The model under review builds one solid part; all positions refer to its coordinate system, in mm. A direction names the side the tool comes from. Coordinates: 2 decimals unless noted, no trailing zeros. Loops run counter-clockwise (first coordinate to the right, second up) from the corner with the lowest first, then second, coordinate; pieces in that order, holes last. Notation, with made-up numbers: M 49.25,-24.75 L 108.25,-24.75 A19 ccw 108.25,-0.75 Z; hole C 57.25,80.25 d6. An arc over 180 degrees is marked long. Use CSV: the item, a comma, the result in double quotes. Start each with the question number.
1. Add section C-C, the plane y = 12.5. Write out the cut boundary in (x, z), then the cut area to 3 significant figures.
2. Tool access review of faces 4 (the cylindrical face through (-68.092, 50.041, 19.399)), 5 (the flat face through (1, 0, 10)), 6 (the flat face through (1, 24, 0)): name each direction out of +Z, -Z, +X, -X, +Y, -Y from which nothing blocks a thin tool from reaching the whole face with its end or side.
3. Add section A-A, the plane z = 34. Write out the cut boundary in (x, y).
4. Clearance check with flat-ended pins moving along their axes: P1, Ø6.5, axis at x = 31.5, z = 20, coming from the -Y side; P2, Ø5, axis at x = 70, z = 20, coming from the -Y side; P3, Ø2.5, axis at x = -70, z = 20, coming from the -Y side. State where each tip first meets the part, or that it passes through.
5. For L1, parallel to Z at x = 80, y = 5; L2, parallel to X at y = 35, z = 36.5; L3, parallel to X at y = 25, z = 20, list the stretches that pass through material, from the lowest coordinate up.
6. Add section B-B, the plane x = -31.5. Write out the cut boundary in (y, z), then the cut area to 3 significant figures.
7. Add section D-D, the plane z = 20. Write out the cut boundary in (x, y), then the cut area to 3 significant figures.
8. Draft analysis for pull direction Z (two halves, no side actions). For faces 1 (the flat face through (1, 25, 40)), 2 (the flat face through (1, -5.303, 5)), 3 (the cylindrical face through (31.17, 34.26, 17.52)), state which applies: +Z half, -Z half, draft (parallel to the pull), parting line (faces both ways), or undercut.
from build123d import *

# Parameters (mm, degrees)
SKETCH1_R                       = 10.75
BOSS_EXTRUDE1_DEPTH             = 40
BOSS_EXTRUDE2_REACH             = 92
BOSS_EXTRUDE2_DIRECTION_2_REACH = 92
SKETCH5_R                       = 2.5
CUT_EXTRUDE1_DEPTH              = 54.696523
CUT_EXTRUDE3_REACH              = 62
SKETCH8_R                       = 2


with BuildPart() as part:
    # Sketch1 → Boss-Extrude1 (new body)
    with BuildSketch(Plane.XY):
        with BuildLine():
            Line((-70, 54.696522502), (70, 54.696522502))
            ThreePointArc((70, 54.696522502), (84.142135624, 48.838658125), (90, 34.696522502))
            Line((90, 34.696522502), (90, 14.696522502))
            Line((90, 14.696522502), (-90, 14.696522502))
            Line((-90, 14.696522502), (-90, 34.696522502))
            ThreePointArc((-90, 34.696522502), (-84.142135624, 48.838658125), (-70, 54.696522502))
        make_face()
        with Locations((70, 34.696522502)):
            Circle(SKETCH1_R, mode=Mode.SUBTRACT)
        with Locations((-70, 34.696522502)):
            Circle(SKETCH1_R, mode=Mode.SUBTRACT)
    extrude(amount=BOSS_EXTRUDE1_DEPTH)

    # Boss-Extrude2: up to this face of the body (flat: up to its plane)
    boss_extrude2_end = Plane(part.part.faces().sort_by_distance((90, 24.696522502, 20))[0])
    # Sketch4 → Boss-Extrude2 (add, up to the picked face)
    with BuildSketch(Plane(origin=(0, 0, 0), x_dir=(0, 0, -1), z_dir=(1, 0, 0)), mode=Mode.PRIVATE) as boss_extrude2_sk1:
        with BuildLine():
            Line((0, -5.303477498), (0, 14.696522502))
            Line((0, 14.696522502), (-20, 14.696522502))
            ThreePointArc((-20, 14.696522502), (-12.928932188, 11.767590313), (-10, 4.696522502))
            Line((-10, 4.696522502), (-10, -5.303477498))
            Line((-10, -5.303477498), (0, -5.303477498))
        make_face()
    boss_extrude2_tool1 = split(extrude(boss_extrude2_sk1.sketch, amount=BOSS_EXTRUDE2_REACH, mode=Mode.PRIVATE), bisect_by=boss_extrude2_end, keep=Keep.BOTH, mode=Mode.PRIVATE)
    add(boss_extrude2_tool1.solids().sort_by_distance((0, 5.449103, 5.700966))[0])
    # Sketch4 → Boss-Extrude2 (add, up to the picked face)
    with BuildSketch(Plane(origin=(0, 0, 0), x_dir=(0, 0, -1), z_dir=(1, 0, 0)), mode=Mode.PRIVATE) as boss_extrude2_sk2:
        with BuildLine():
            ThreePointArc((-30, 4.696522502), (-27.071067812, 11.767590313), (-20, 14.696522502))
            Line((-20, 14.696522502), (-40, 14.696522502))
            Line((-40, 14.696522502), (-40, -5.303477498))
            Line((-40, -5.303477498), (-30, -5.303477498))
            Line((-30, -5.303477498), (-30, 4.696522502))
        make_face()
    boss_extrude2_tool2 = split(extrude(boss_extrude2_sk2.sketch, amount=BOSS_EXTRUDE2_REACH, mode=Mode.PRIVATE), bisect_by=boss_extrude2_end, keep=Keep.BOTH, mode=Mode.PRIVATE)
    add(boss_extrude2_tool2.solids().sort_by_distance((0, 5.449103, 34.299034))[0])

    # Boss-Extrude2 direction 2: up to this face of the body (flat: up to its plane)
    boss_extrude2_direction_2_end = Plane(part.part.faces().sort_by_distance((-90, 24.696522502, 20))[0])
    # Sketch4 → Boss-Extrude2 direction 2 (add, up to the picked face)
    with BuildSketch(Plane(origin=(0, 0, 0), x_dir=(0, 0, -1), z_dir=(1, 0, 0)), mode=Mode.PRIVATE) as boss_extrude2_direction_2_sk1:
        with BuildLine():
            Line((0, -5.303477498), (0, 14.696522502))
            Line((0, 14.696522502), (-20, 14.696522502))
            ThreePointArc((-20, 14.696522502), (-12.928932188, 11.767590313), (-10, 4.696522502))
            Line((-10, 4.696522502), (-10, -5.303477498))
            Line((-10, -5.303477498), (0, -5.303477498))
        make_face()
    boss_extrude2_direction_2_tool1 = split(extrude(boss_extrude2_direction_2_sk1.sketch, amount=-BOSS_EXTRUDE2_DIRECTION_2_REACH, mode=Mode.PRIVATE), bisect_by=boss_extrude2_direction_2_end, keep=Keep.BOTH, mode=Mode.PRIVATE)
    add(boss_extrude2_direction_2_tool1.solids().sort_by_distance((0, 5.449103, 5.700966))[0])
    # Sketch4 → Boss-Extrude2 direction 2 (add, up to the picked face)
    with BuildSketch(Plane(origin=(0, 0, 0), x_dir=(0, 0, -1), z_dir=(1, 0, 0)), mode=Mode.PRIVATE) as boss_extrude2_direction_2_sk2:
        with BuildLine():
            ThreePointArc((-30, 4.696522502), (-27.071067812, 11.767590313), (-20, 14.696522502))
            Line((-20, 14.696522502), (-40, 14.696522502))
            Line((-40, 14.696522502), (-40, -5.303477498))
            Line((-40, -5.303477498), (-30, -5.303477498))
            Line((-30, -5.303477498), (-30, 4.696522502))
        make_face()
    boss_extrude2_direction_2_tool2 = split(extrude(boss_extrude2_direction_2_sk2.sketch, amount=-BOSS_EXTRUDE2_DIRECTION_2_REACH, mode=Mode.PRIVATE), bisect_by=boss_extrude2_direction_2_end, keep=Keep.BOTH, mode=Mode.PRIVATE)
    add(boss_extrude2_direction_2_tool2.solids().sort_by_distance((0, 5.449103, 34.299034))[0])

    # Sketch5 → Cut-Extrude1 (cut)
    with BuildSketch(Plane(origin=(0, 0, 0), x_dir=(1, 0, 0), z_dir=(0, 1, 0))):
        with Locations((-31.5, -20)):
            Circle(SKETCH5_R)
        with Locations((31.5, -20)):
            Circle(SKETCH5_R)
    extrude(amount=CUT_EXTRUDE1_DEPTH, mode=Mode.SUBTRACT)

    # Sketch8 → Cut-Extrude3 (cut, up to next)
    with BuildSketch(Plane(origin=(0, 54.696522502, 0), x_dir=(1, 0, 0), z_dir=(0, 1, 0)), mode=Mode.PRIVATE) as cut_extrude3_sk1:
        with Locations((-70, -20)):
            Circle(SKETCH8_R)
    cut_extrude3_tool1 = extrude(cut_extrude3_sk1.sketch, amount=-CUT_EXTRUDE3_REACH, mode=Mode.PRIVATE) & part.part
    add(cut_extrude3_tool1.solids().sort_by_distance((-70, 54.696523, 20))[0], mode=Mode.SUBTRACT)
    # Sketch8 → Cut-Extrude3 (cut, up to next)
    with BuildSketch(Plane(origin=(0, 54.696522502, 0), x_dir=(1, 0, 0), z_dir=(0, 1, 0)), mode=Mode.PRIVATE) as cut_extrude3_sk2:
        with Locations((70, -20)):
            Circle(SKETCH8_R)
    cut_extrude3_tool2 = extrude(cut_extrude3_sk2.sketch, amount=-CUT_EXTRUDE3_REACH, mode=Mode.PRIVATE) & part.part
    add(cut_extrude3_tool2.solids().sort_by_distance((70, 54.696523, 20))[0], mode=Mode.SUBTRACT)


solid = part.part
Computed:
1,outline,"M -90,0 L 90,0 L 90,13.75 L -90,13.75 Z; M -90,26.25 L 90,26.25 L 90,40 L -90,40 Z"
1,area,"4,950 mm^2"
2,face 4,"+Y"
2,face 5,"+X, -X, -Y"
2,face 6,"-Z, +X, -X, +Y, -Y"
3,outline,"M -90,-5.3 L 90,-5.3 L 90,34.7 A20 ccw 70,54.7 L -70,54.7 A20 ccw -90,34.7 Z; hole C -70,34.7 d21.5; hole C 70,34.7 d21.5"
4,P1,"stops at y = 14.15"
4,P2,"stops at y = 14.38"
4,P3,"stops at y = 14.62"
5,L1,"z = 0 to 10, 30 to 40"
5,L2,"x = -90 to -80.75, -59.25 to 59.25, 80.75 to 90"
5,L3,"x = -90 to -74.64, -65.36 to -34, -29 to 29, 34 to 65.36, 74.64 to 90"
6,outline,"M -5.3,0 L 54.7,0 L 54.7,17.5 L 14.38,17.5 A10 cw 4.7,10 L -5.3,10 Z; M -5.3,30 L 4.7,30 A10 cw 14.38,22.5 L 54.7,22.5 L 54.7,40 L -5.3,40 Z"
6,area,"1,840 mm^2"
7,outline,"M -90,14.7 L -34,14.7 L -34,54.7 L -68,54.7 L -68,45.26 A10.75 cw long -72,45.26 L -72,54.6 A20 ccw -90,34.7 Z; M -29,14.7 L 29,14.7 L 29,54.7 L -29,54.7 Z; M 34,14.7 L 90,14.7 L 90,34.7 A20 ccw 72,54.6 L 72,45.26 A10.75 cw long 68,45.26 L 68,54.7 L 34,54.7 Z"
7,area,"5,830 mm^2"
8,face 1,"+Z half"
8,face 2,"draft"
8,face 3,"undercut"
